from build123d import *

# Parameters (mm, degrees)
SKETCH_1_R          = 1.5
EXTRUDE_1_DEPTH     = 1.5
EXTRUDE_1_2_DEPTH   = 1.5
EXTRUDE_1_3_DEPTH   = 1.5
SKETCH_1_W          = 5.434310226
SKETCH_1_H          = 3.069112814
EXTRUDE_1_4_DEPTH   = 1.5
SKETCH_1_W_2        = 2.364591514
SKETCH_1_H_2        = 3.137743857
EXTRUDE_1_5_DEPTH   = 1.5
EXTRUDE_2_DEPTH     = 1.5
SKETCH_5_W          = 28.57510237
SKETCH_5_H          = 2.837891342
SKETCH_5_W_2        = 23.917529704
SKETCH_5_H_2        = 1.634820582
EXTRUDE_3_DEPTH     = 4.1
SKETCH_6_W          = 0.787454543
SKETCH_6_H          = 7.1
EXTRUDE_4_DEPTH     = 2.837891342
EXTRUDE_5_DEPTH     = 15.344031237
CUT_EXTRUDE_1_DEPTH = 4.1
EXTRUDE_6_DEPTH     = 1.634820582
EXTRUDE_7_REACH     = 88.228
SKETCH_10_W         = 6.524128353
SKETCH_10_H         = 3


with BuildPart() as part:
    # Sketch 1 → Extrude 1 (new body)
    with BuildSketch(Plane.XY):
        with BuildLine():
            Line((42.374172917, 38.777020574), (73.737536195, 38.777020574))
            ThreePointArc((73.737536195, 38.777020574), (75.829099502, 37.910666686), (76.695453391, 35.819103378))
            Line((76.695453391, 35.819103378), (76.695453391, 2.836372873))
            ThreePointArc((76.695453391, 2.836372873), (75.868418762, 0.839734655), (73.871780544, 0.012700025))
            Line((73.871780544, 0.012700025), (65.856491688, 0.012700025))
            Line((65.856491688, 0.012700025), (65.856491688, 13.044712807))
            Line((65.856491688, 13.044712807), (70.100741351, 13.044712807))
            Line((70.100741351, 13.044712807), (70.100741351, 20.05420005))
            Line((70.100741351, 20.05420005), (44.751683648, 20.05420005))
            Line((44.751683648, 20.05420005), (44.751683648, 16.790663202))
            Line((44.751683648, 16.790663202), (30.415811039, 16.790663202))
            Line((30.415811039, 16.790663202), (30.415811039, 26.437124649))
            Line((30.415811039, 26.437124649), (36.705891976, 26.437124649))
            Line((36.705891976, 26.437124649), (36.705891976, 22.429523721))
            Line((36.705891976, 22.429523721), (44.751683648, 22.429523721))
            Line((44.751683648, 22.429523721), (44.751683648, 32.470424916))
            Line((44.751683648, 32.470424916), (42.374172917, 32.470424916))
            Line((42.374172917, 32.470424916), (42.374172917, 38.777020574))
        make_face()
        with Locations((73.871780544, 2.882016764)):
            Circle(SKETCH_1_R, mode=Mode.SUBTRACT)
        with Locations((73.871780544, 35.894081788)):
            Circle(SKETCH_1_R, mode=Mode.SUBTRACT)
    extrude(amount=EXTRUDE_1_DEPTH)



with BuildPart() as body_2:
    # Sketch 1 → Extrude 1 2 (new body)
    with BuildSketch(Plane.XY):
        with BuildLine():
            Line((20.832405991, 0.012700025), (2.882016764, 0.012700025))
            ThreePointArc((2.882016764, 0.012700025), (0.853103441, 0.853103441), (0.012700025, 2.882016764))
            Line((0.012700025, 2.882016764), (0.012700025, 16.410813367))
            Line((0.012700025, 16.410813367), (3.46840969, 16.410813367))
            Line((3.46840969, 16.410813367), (3.46840969, 7.290825892))
            Line((3.46840969, 7.290825892), (6.394972835, 5.203664579))
            Line((6.394972835, 5.203664579), (6.394972835, 1.925003773))
            Line((6.394972835, 1.925003773), (14.41516881, 1.925003773))
            Line((14.41516881, 1.925003773), (14.41516881, 1.467481791))
            Line((14.41516881, 1.467481791), (20.832405991, 1.467481791))
            Line((20.832405991, 1.467481791), (33.595883095, 1.467481791))
            Line((33.595883095, 1.467481791), (33.595883095, 4.637617134))
            Line((33.595883095, 4.637617134), (40.626678312, 4.637617134))
            Line((40.626678312, 4.637617134), (40.626678312, 0.012700025))
            Line((40.626678312, 0.012700025), (33.595883095, 0.012700025))
            Line((33.595883095, 0.012700025), (20.832405991, 0.012700025))
        make_face()
        with Locations((2.902413005, 2.882016764)):
            Circle(SKETCH_1_R, mode=Mode.SUBTRACT)
    extrude(amount=EXTRUDE_1_2_DEPTH)


with BuildPart() as body_3:
    # Sketch 1 → Extrude 1 3 (new body)
    with BuildSketch(Plane.XY):
        with BuildLine():
            Line((2.857505715, 38.777020574), (26.242687137, 38.777020574))
            Line((26.242687137, 38.777020574), (26.242687137, 30.345137506))
            Line((26.242687137, 30.345137506), (2.385627897, 30.345137506))
            Line((2.385627897, 30.345137506), (2.385627897, 30.834185958))
            Line((2.385627897, 30.834185958), (0.012700025, 30.834185958))
            Line((0.012700025, 30.834185958), (0.012700025, 35.932214884))
            ThreePointArc((0.012700025, 35.932214884), (0.845924321, 37.943796279), (2.857505715, 38.777020574))
        make_face()
        with Locations((2.857505715, 35.877571755)):
            Circle(SKETCH_1_R, mode=Mode.SUBTRACT)
    extrude(amount=EXTRUDE_1_3_DEPTH)


with BuildPart() as body_4:
    # Sketch 1 → Extrude 1 4 (new body)
    with BuildSketch(Plane.XY):
        with Locations((45.09132803, 11.774429054)):
            Rectangle(SKETCH_1_W, SKETCH_1_H)
    extrude(amount=EXTRUDE_1_4_DEPTH)


with BuildPart() as body_5:
    # Sketch 1 → Extrude 1 5 (new body)
    with BuildSketch(Plane.XY):
        with Locations((48.333102422, 1.581571954)):
            Rectangle(SKETCH_1_W_2, SKETCH_1_H_2)
    extrude(amount=EXTRUDE_1_5_DEPTH)


with BuildPart() as part_1:
    add(part.part)

    add(body_2.part)  # Extrude 2 merges body 2

    add(body_3.part)  # Extrude 2 merges body 3

    add(body_4.part)  # Extrude 2 merges body 4

    add(body_5.part)  # Extrude 2 merges body 5
    # Sketch 3 → Extrude 2 (add)
    with BuildSketch(Plane.XY.offset(1.5)):
        Polygon((0.012700025, 34.205237949), (0.012700025, 30.834185958), (0.012700025, 23.817436756), (2.385627897, 23.817436756), (2.385627897, 30.345137506), (26.242687137, 30.345137506), (26.242687137, 38.777020574), (5.701940925, 38.777020574), (5.701940925, 34.225848847), (2.857505715, 32.577891407), align=None)
        Polygon((42.374172917, 38.777020574), (70.949275287, 38.777020574), (70.949275287, 34.225848847), (73.852441207, 32.577891407), (76.695453391, 34.225848847), (76.695453391, 4.574174261), (73.852441207, 6.187985945), (71.068336369, 4.574174261), (71.068336369, 0.012700025), (65.856491688, 0.012700025), (65.856491688, 13.044712807), (65.856491688, 15.972548736), (47.813055626, 15.972548736), (47.808483143, 13.308985461), (47.808483143, 3.150443882), (49.515398179, 3.150443882), (49.515398179, 0.012700025), (47.150806665, 0.012700025), (47.150806665, 5.096192633), (42.374172917, 5.096192633), (40.626678312, 5.096192633), (40.626678312, 4.637617134), (40.626678312, 0.012700025), (40.056713733, 0.012700025), (5.783059857, 0.012700025), (5.783059857, 4.506035797), (2.882016764, 6.187985945), (0.012700025, 4.506035797), (0.012700025, 16.410813367), (3.46840969, 16.410813367), (3.46840969, 14.453016608), (6.394972835, 14.453016608), (6.394972835, 10.104845947), (6.394972835, 5.203664579), (6.394972835, 1.925003773), (13.068362142, 1.925003773), (13.068362142, 3.23686167), (20.727981914, 3.23686167), (20.727981914, 23.163322327), (30.415811039, 23.163322327), (30.415811039, 26.437124649), (36.705891976, 26.437124649), (36.705891976, 22.429523721), (42.374172917, 22.429523721), align=None)
    extrude(amount=EXTRUDE_2_DEPTH)

    # Sketch 5 → Extrude 3 (add)
    with BuildSketch(Plane.XY.offset(3)):
        with Locations((56.661724102, 37.358074903)):
            Rectangle(SKETCH_5_W, SKETCH_5_H)
        Polygon((76.695453391, 34.225848847), (73.852441207, 32.577891407), (71.189142318, 34.089690367), (71.189142318, 4.64419966), (73.852441207, 6.187985945), (76.695453391, 4.574174261), align=None)
        with Locations((59.109571517, 0.830110316)):
            Rectangle(SKETCH_5_W_2, SKETCH_5_H_2)
        Polygon((40.626678312, 0.012700025), (6.394972835, 0.012700025), (5.783059857, 0.012700025), (5.783059857, 4.506035797), (2.882016764, 6.187985945), (0.012700025, 4.506035797), (0.012700025, 16.410813367), (0.012700025, 23.817436756), (0.012700025, 34.205237949), (2.857505715, 32.577891407), (5.701940925, 34.225848847), (5.701940925, 38.777020574), (26.242687137, 38.777020574), (26.242687137, 35.939129232), (20.953318595, 35.939129232), (20.953318595, 30.345137506), (2.385627897, 30.345137506), (2.385627897, 23.817436756), (2.385627897, 16.410813367), (3.46840969, 16.410813367), (3.46840969, 14.453016608), (6.394972835, 14.453016608), (6.394972835, 1.925003773), (13.068362142, 1.925003773), (13.068362142, 3.23686167), (20.727981914, 3.23686167), (20.727981914, 1.423006096), (40.626678312, 1.423006096), align=None)
    extrude(amount=EXTRUDE_3_DEPTH)

    # Sketch 6 → Extrude 4 (add)
    with BuildSketch(Plane(origin=(0, 38.777020574, 0), x_dir=(1, 0, 0), z_dir=(0, 1, 0))):
        with Locations((41.980445645, -3.55)):
            Rectangle(SKETCH_6_W, SKETCH_6_H)
    extrude(amount=-EXTRUDE_4_DEPTH)

    # Sketch 7 → Extrude 5 (add)
    with BuildSketch(Plane.ZY.offset(-41.586718374)):
        with BuildLine():
            Line((7.1, 35.939129232), (2.269100337, 35.939129232))
            Line((2.269100337, 35.939129232), (2.269100337, 37.022377445))
            ThreePointArc((2.269100337, 37.022377445), (2.47412559, 37.517352192), (2.969100337, 37.722377445))
            Line((2.969100337, 37.722377445), (7.1, 37.722377445))
            Line((7.1, 37.722377445), (7.1, 35.939129232))
        make_face()
    extrude(amount=EXTRUDE_5_DEPTH)

    # Sketch 8 → Cut-Extrude 1 (cut)
    with BuildSketch(Plane.XY.offset(7.1)):
        with BuildLine():
            Line((20.953318595, 35.939129232), (15.992068639, 35.939129232))
            ThreePointArc((15.992068639, 35.939129232), (14.486042091, 35.31531261), (13.862225469, 33.809286062))
            Line((13.862225469, 33.809286062), (13.862225469, 30.345137506))
            Line((13.862225469, 30.345137506), (15.632095679, 30.345137506))
            Line((15.632095679, 30.345137506), (15.632095679, 33.321819521))
            ThreePointArc((15.632095679, 33.321819521), (15.872616168, 33.902487347), (16.453283994, 34.143007835))
            Line((16.453283994, 34.143007835), (20.953318595, 34.143007835))
            Line((20.953318595, 34.143007835), (20.953318595, 35.939129232))
        make_face()
    extrude(amount=-CUT_EXTRUDE_1_DEPTH, mode=Mode.SUBTRACT)

    # Sketch 9 → Extrude 6 (add)
    with BuildSketch(Plane.XZ.offset(-0.012700025)):
        Polygon((49.515398179, 2.203775642), (64.615113945, 2.203775642), (64.615113945, 0), (65.856491688, 0), (65.856491688, 3), (49.515398179, 3), align=None)
    extrude(amount=-EXTRUDE_6_DEPTH)

    # Extrude 7: up to this face of the body (flat: up to its plane)
    extrude_7_end = Plane(part_1.part.faces().sort_by_distance((59.094076967, 1.647520607, 4.675215674))[0])
    # Sketch 10 → Extrude 7 (add, up to the picked face)
    with BuildSketch(Plane.XZ.offset(-0.012700025), mode=Mode.PRIVATE) as extrude_7_sk1:
        with Locations((43.888742489, 5.6)):
            Rectangle(SKETCH_10_W, SKETCH_10_H)
    extrude_7_tool1 = split(extrude(extrude_7_sk1.sketch, amount=-EXTRUDE_7_REACH, mode=Mode.PRIVATE), bisect_by=extrude_7_end, keep=Keep.BOTH, mode=Mode.PRIVATE)
    add(extrude_7_tool1.solids().sort_by(Axis((43.888742, 0.0127, 5.6), (0, 1, 0)))[0])


solid = part_1.part
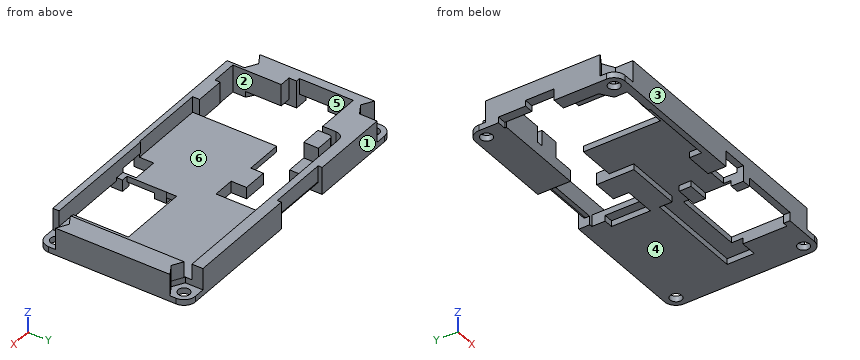
Can you work these out from the model? Positions are in its coordinate system, mm. Face numbers are marked on the shaded views. A direction names the side the tool comes from. Give positions to 0.01 mm unless a question says otherwise; leave off trailing zeros. Loops run counter-clockwise (first coordinate to the right, second up) from the corner with the lowest first, then second, coordinate; pieces in that order, holes last. Notation, with made-up numbers: (53, 30) -> (70, 30) arc R20 cw to (70, 34) -> close; hole circle Ø2 at (-32, 86). An arc over 180 degrees is marked (long way). Write item = value, one per line.
1) Suppose I cut it at B-B on y = 9.5. Write out the boundary of the cut face in (x, z), then the cut area to 3 significant figures.
Check result:
outline = (0.01, 0) -> (3.47, 0) -> (3.47, 1.5) -> (6.39, 1.5) -> (6.39, 7.1) -> (0.01, 7.1) -> close; (20.73, 1.5) -> (47.81, 1.5) -> (47.81, 3) -> (20.73, 3) -> close; (65.86, 0) -> (76.7, 0) -> (76.7, 7.1) -> (71.19, 7.1) -> (71.19, 3) -> (65.86, 3) -> close
area = 137 mm2
2) I need wall thicknesses on L1, parallel to Y at x = 16.5, z = 4.75; L2, parallel to Y at x = 60, z = 2.25; L3, parallel to X at y = 11.5, z = 1.75. Which ranges of each line are inside material? Lowest first, please. Write a range as from..to.
Check result:
L1 = 0.01..3.24, 30.35..34.14, 35.94..38.78
L2 = 0.01..1.65, 15.97..38.78
L3 = 0.01..6.39, 20.73..47.81, 65.86..76.7
3) Suppose I cut it at D-D on x = 24. Write out the boundary of the cut face in (y, z).
Check result:
outline = (0.01, 0) -> (1.47, 0) -> (1.47, 1.5) -> (23.16, 1.5) -> (23.16, 3) -> (1.42, 3) -> (1.42, 7.1) -> (0.01, 7.1) -> close; (30.35, 0) -> (38.78, 0) -> (38.78, 7.1) -> (35.94, 7.1) -> (35.94, 3) -> (30.35, 3) -> close
4) Suppose I cut it at A-A on x = 61. Write out the boundary of the cut face in (y, z), then the cut area to 3 significant figures.
Check result:
outline = (0.01, 2.2) -> (1.65, 2.2) -> (1.65, 7.1) -> (0.01, 7.1) -> close; (15.97, 1.5) -> (20.05, 1.5) -> (20.05, 0) -> (38.78, 0) -> (38.78, 7.1) -> (35.94, 7.1) -> (35.94, 3) -> (15.97, 3) -> close
area = 81.9 mm2
5) Suppose I cut it at C-C on y = 29.5. Write out the boundary of the cut face in (x, z), then the cut area to 3 significant figures.
Check result:
outline = (0.01, 1.5) -> (2.39, 1.5) -> (2.39, 7.1) -> (0.01, 7.1) -> close; (42.37, 1.5) -> (44.75, 1.5) -> (44.75, 0) -> (76.7, 0) -> (76.7, 7.1) -> (71.19, 7.1) -> (71.19, 3) -> (42.37, 3) -> close
area = 135 mm2
6) For the marked faces 4, 5 and 6, which set-ups out of +Z, -Z, +X, -X, +Y, -Y let a thin tool reach every point of the face, with its end or its side?
Check result:
face_4 = -Z, +X, -X, +Y, -Y
face_5 = +Z, -Z
face_6 = +Z
7) Thinking about a two-plate mould opening in Y: for the marked faces 1, 2 and 3, which applies, released by +Y, released by -Y, zero draft, split by the parting line, or undercut?
Check result:
face_1 = released by +Y
face_2 = undercut
face_3 = released by -Y
8) Will these pins go through, and if not, where does the flat tip stop? pin 1 (1.4 mm diameter, centred on y = 2.5, z = 5, fed in from -X); pin 2 (3 mm diameter, centred on x = 73.5, y = 3.5, fed in from +Z); pin 3 (8 mm diameter, centred on x = 38.5, y = 25.5, fed in from +Z).
Check result:
pin_1 = 5.78
pin_2 = 1.5
pin_3 = 3
